Design review of the part built by this model. Coordinates are the model's own, in mm. A direction names the side the tool comes from. Round coordinates to 2 decimals unless told otherwise and drop trailing zeros. Order: outer loops, then holes, each group sorted by start corner. A loop starts at its lowest first (then second) coordinate and runs counter-clockwise, first axis right, second up. Notation, with made-up numbers: (11, 71) - (24, 71) arc R14 cw to (24, 84) - close; hole circle Ø6 at (-0.5, -3). An arc over 180 degrees is marked (long way). Write item = value, one per line.
from build123d import *

# Parameters (mm, degrees)
SKETCH2_W                            = 31.75
SKETCH2_H                            = 38.1
BASE_FLANGE1_DEPTH                   = 2.54
EDGE_FLANGE2_DEPTH                   = 38.1
EDGE_FLANGE2_BEND_DEPTH              = 38.1
F_21_64_0_32813_DIAMETER_HOLE1_D     = 8.334502
F_21_64_0_32813_DIAMETER_HOLE1_DEPTH = 25.4
F_21_64_0_32813_DIAMETER_HOLE1_TIP   = 2.503937016
F_21_64_0_32813_DIAMETER_HOLE2_D     = 8.334502


# Sheet-metal steps are written as plain solids
with BuildPart() as part:
    # Sketch2 → Base-Flange1 (new body)
    with BuildSketch(Plane.XY):
        Rectangle(SKETCH2_W, SKETCH2_H)
    extrude(amount=-BASE_FLANGE1_DEPTH)

    # Edge-Flange2 section (across the edge) → Edge-Flange2 (add)
    with BuildSketch(Plane(origin=(19.05, 19.05, -2.54), x_dir=(-1, 0, 0), z_dir=(0, -1, 0))):
        with BuildLine():
            Line((-2.54, 3.175), (-2.54, 34.29))
            Line((-2.54, 34.29), (0, 34.29))
            Line((0, 34.29), (0, 3.175))
            ThreePointArc((0, 3.175), (0.92993597, 0.92993597), (3.175, 0))
            Line((3.175, 0), (3.175, -2.54))
            ThreePointArc((3.175, -2.54), (-0.866115254, -0.866115254), (-2.54, 3.175))
        make_face()
    extrude(amount=EDGE_FLANGE2_DEPTH)

    # Edge-Flange2 section 2 (across the edge) → Edge-Flange2 bend (add)
    with BuildSketch(Plane(origin=(-19.05, -19.05, -2.54), x_dir=(1, 0, 0), z_dir=(0, 1, 0))):
        with BuildLine():
            Line((-2.54, 3.175), (-2.54, 34.29))
            Line((-2.54, 34.29), (0, 34.29))
            Line((0, 34.29), (0, 3.175))
            ThreePointArc((0, 3.175), (0.92993597, 0.92993597), (3.175, 0))
            Line((3.175, 0), (3.175, -2.54))
            ThreePointArc((3.175, -2.54), (-0.866115254, -0.866115254), (-2.54, 3.175))
        make_face()
    extrude(amount=EDGE_FLANGE2_BEND_DEPTH)

    # 21/64 (0.32813) Diameter Hole1
    with Locations(Plane.XY):
        with Locations((0, 0)):
            Hole(F_21_64_0_32813_DIAMETER_HOLE1_D / 2, depth=F_21_64_0_32813_DIAMETER_HOLE1_DEPTH)
            with Locations((0, 0, -(F_21_64_0_32813_DIAMETER_HOLE1_DEPTH + F_21_64_0_32813_DIAMETER_HOLE1_TIP / 2))):  # 118° drill point
                Cone(0, F_21_64_0_32813_DIAMETER_HOLE1_D / 2, F_21_64_0_32813_DIAMETER_HOLE1_TIP, mode=Mode.SUBTRACT)

    # 21/64 (0.32813) Diameter Hole2 (through all)
    with Locations(Plane(origin=(21.59, 0, 0), x_dir=(0, 0, -1), z_dir=(1, 0, 0))):
        with Locations((21.2725, 0)):
            Hole(F_21_64_0_32813_DIAMETER_HOLE2_D / 2)


solid = part.part
Item 1: The part is to be moulded in two halves that separate along Z. For faces 1 (the face through (-20, 0, -36.83)), 2 (the face through (-19.05, -5, -21)), 3 (the face through (-20.338, 0.183, -25.436)), say which applies: +Z half, -Z half, draft (parallel to the pull), parting line (faces both ways), or undercut.
Data:
face_1 = -Z half
face_2 = draft
face_3 = undercut
Item 2: For line 1 along Y through (x, z) = (0, -1.9); line 2 along X through (y, z) = (-13, -20.5); line 3 along Z through (x, y) = (-9, 10), list the stretches that pass through material, from the lowest coordinate up. Write a range as [from, to].
Data:
line_1 = [-19.05, -4.17], [4.17, 19.05]
line_2 = [-21.59, -19.05], [19.05, 21.59]
line_3 = [-2.54, 0]
Item 3: Take a section at D-D, the plane x = -11. State the section outline as (y, z) points, and give its area (3 significant figures).
Data:
outline = (-19.05, -2.54) - (19.05, -2.54) - (19.05, 0) - (-19.05, 0) - close
area = 96.8 mm2
Item 4: Take a section at C-C, the plane y = 5. State the section outline as (x, z) points (3 decimals), and give its area (3 significant figures).
Data:
outline = (-21.59, -36.83) - (-19.05, -36.83) - (-19.05, -5.715) arc R3.175 cw to (-15.875, -2.54) - (15.875, -2.54) arc R3.175 cw to (19.05, -5.715) - (19.05, -36.83) - (21.59, -36.83) - (21.59, -5.715) arc R5.715 ccw to (15.875, 0) - (-15.875, 0) arc R5.715 ccw to (-21.59, -5.715) - close
area = 274 mm2
Item 5: Insertion check: P1, Ø9.5, axis at x = -7.5, y = 2.5, coming from the -Z side; P2, Ø5, axis at y = 0, z = -21.27, coming from the -X side. Each pin has a flat end and moves straight along its axis. Give the tip position at first contact, or say it passes through.
Data:
P1 = -2.54
P2 = through
Item 6: Take a section at B-B, the plane z = -26.5. State the section outline as (x, y) points.
Data:
outline = (-21.59, -19.05) - (-19.05, -19.05) - (-19.05, 19.05) - (-21.59, 19.05) - close; (19.05, -19.05) - (21.59, -19.05) - (21.59, 19.05) - (19.05, 19.05) - close
Item 7: Take a section at A-A, the plane y = 0. State the section outline as (x, z) points (3 decimals).
Data:
outline = (-21.59, -36.83) - (-19.05, -36.83) - (-19.05, -25.44) - (-21.59, -25.44) - close; (-21.59, -17.105) - (-19.05, -17.105) - (-19.05, -5.715) arc R3.175 cw to (-15.875, -2.54) - (-4.167, -2.54) - (-4.167, 0) - (-15.875, 0) arc R5.715 ccw to (-21.59, -5.715) - close; (4.167, -2.54) - (15.875, -2.54) arc R3.175 cw to (19.05, -5.715) - (19.05, -17.105) - (21.59, -17.105) - (21.59, -5.715) arc R5.715 ccw to (15.875, 0) - (4.167, 0) - close; (19.05, -36.83) - (21.59, -36.83) - (21.59, -25.44) - (19.05, -25.44) - close
Item 8: For faces 4 (the face through (20, 0, -36.83)), 5 (the face through (-18.14, -0.27, -3.49)), list the 3-axis set-ups (+Z, -Z, +X, -X, +Y, -Y) from which the entire face can be reached by the end or side of a thin tool; tool diameter is ignored.
Data:
face_4 = -Z, +X, -X, +Y, -Y
face_5 = -Z, +Y, -Y
